Work out the finished part from the listing and answer in its coordinate system (mm). Coordinates: 2 decimals unless noted, no trailing zeros. Write each loop counter-clockwise with the first axis right and the second up, starting at its lowest first coordinate (ties: lowest second). Pieces come first, ordered by that corner, then holes. Notation, with made-up numbers: (8, 39.25) - (19, 39.25) arc R21 ccw to (19, 75.25) - close; hole circle Ø7 at (80.25, 13). An arc over 180 degrees is marked (long way). Use one line per item in the form item = value. Start each with the question number.
Item 1: A cutting plane is placed at A-A (x = 58). Write down the section's boundary in (y, z), then the cut area to 3 significant figures.
Item 2: Consider probe 1 along Y at (x, z) = (79.5, 1.2); probe 2 along X at (y, z) = (-79.5, 2.4). Determine where each line is inside the solid, lowest interval first.
Item 3: Given pin 1 (1.5 mm diameter, centred on y = -182.5, z = 1.5, fed in from +X); pin 2 (5 mm diameter, centred on x = 23.5, y = -158, fed in from -Z); pin 3 (0.9 mm diameter, centred on x = 81, z = 1, fed in from -Y); pin 4 (1.5 mm diameter, centred on x = 55, z = 1.5, fed in from +Y), each flat-ended and moving along its own axis, determine where each tip first touches the part or whether it passes through.
from build123d import *

# Parameters (mm, degrees)
ESQUISSE1_W                = 80
ESQUISSE1_H                = 189.15
BOSS_EXTRU_1_DEPTH         = 3
ESQUISSE3_W                = 10
ESQUISSE3_H                = 3
BOSS_EXTRU_2_DEPTH         = 3
R_P_TITION_LIN_AIRE1_COUNT = 4
R_P_TITION_LIN_AIRE1_PITCH = 20
ESQUISSE4_W                = 10
ESQUISSE4_H                = 3
BOSS_EXTRU_3_DEPTH         = 3
R_P_TITION_LIN_AIRE2_COUNT = 4
R_P_TITION_LIN_AIRE2_PITCH = 20
ESQUISSE5_W                = 3
ESQUISSE5_H                = 10
BOSS_EXTRU_4_DEPTH         = 3
R_P_TITION_LIN_AIRE3_COUNT = 9
R_P_TITION_LIN_AIRE3_PITCH = 20


with BuildPart() as part:
    # Esquisse1 → Boss.-Extru.1 (new body)
    with BuildSketch(Plane.XY):
        with Locations((40, -94.575)):
            Rectangle(ESQUISSE1_W, ESQUISSE1_H)
    extrude(amount=BOSS_EXTRU_1_DEPTH)

    # Esquisse3 → Boss.-Extru.2 (add)
    with BuildSketch(Plane(origin=(0, 0, 0), x_dir=(1, 0, 0), z_dir=(0, 1, 0))):
        with Locations((5, -1.5)):
            Rectangle(ESQUISSE3_W, ESQUISSE3_H)
    boss_extru_2 = extrude(amount=BOSS_EXTRU_2_DEPTH)

    # Répétition linéaire1: Boss.-Extru.2 ×4
    with Locations(*[(i * R_P_TITION_LIN_AIRE1_PITCH, 0, 0) for i in range(1, R_P_TITION_LIN_AIRE1_COUNT)]):
        add(boss_extru_2)

    # Esquisse4 → Boss.-Extru.3 (add)
    with BuildSketch(Plane.XZ.offset(189.15)):
        with Locations((5, 1.5)):
            Rectangle(ESQUISSE4_W, ESQUISSE4_H)
    boss_extru_3 = extrude(amount=BOSS_EXTRU_3_DEPTH)

    # Répétition linéaire2: Boss.-Extru.3 ×4
    with Locations(*[(i * R_P_TITION_LIN_AIRE2_PITCH, 0, 0) for i in range(1, R_P_TITION_LIN_AIRE2_COUNT)]):
        add(boss_extru_3)

    # Esquisse5 → Boss.-Extru.4 (add)
    with BuildSketch(Plane(origin=(80, 0, 0), x_dir=(0, 0, -1), z_dir=(1, 0, 0))):
        with Locations((-1.5, -174.15)):
            Rectangle(ESQUISSE5_W, ESQUISSE5_H)
    boss_extru_4 = extrude(amount=BOSS_EXTRU_4_DEPTH)

    # Répétition linéaire3: Boss.-Extru.4 ×9
    with Locations(*[(0, i * R_P_TITION_LIN_AIRE3_PITCH, 0) for i in range(1, R_P_TITION_LIN_AIRE3_COUNT)]):
        add(boss_extru_4)


solid = part.part
Answer:
q1.outline = (-189.15, 0) - (0, 0) - (0, 3) - (-189.15, 3) - close
q1.area = 567 mm²
q2.probe_1 = -189.15 to 0
q2.probe_2 = 0 to 80
q3.pin_1 = 80
q3.pin_2 = 0
q3.pin_3 = -179.15
q3.pin_4 = 0
